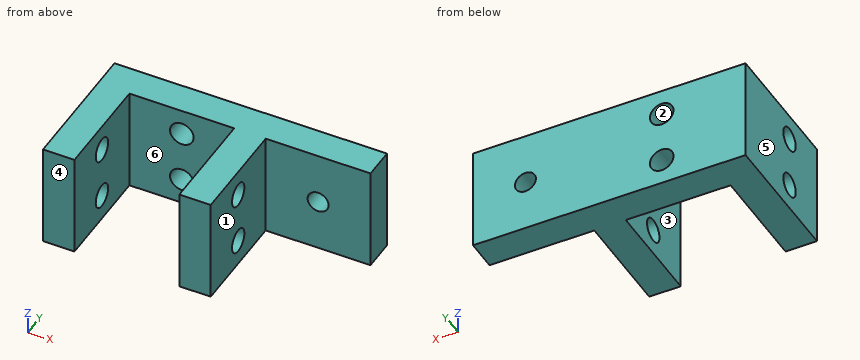
from build123d import *

# Parameters (mm, degrees)
BOSS_EXTRUDE3_DEPTH     = 20
SKETCH9_R               = 2.25
CUT_EXTRUDE1_DEPTH      = 47
CUT_EXTRUDE1_DEPTH_BACK = 7
SKETCH10_R              = 2.25
CUT_EXTRUDE2_DEPTH      = 21
CUT_EXTRUDE2_DEPTH_BACK = 7
SKETCH11_R              = 2
CUT_EXTRUDE3_DEPTH      = 21
CUT_EXTRUDE3_DEPTH_BACK = 7


with BuildPart() as part:
    # Sketch7 → Boss-Extrude3 (new body)
    with BuildSketch(Plane.XY):
        Polygon((-52, -26), (-52, 0), (0, 0), (0, -6), (-20, -6), (-20, -26), (-26, -26), (-26, -6), (-46, -6), (-46, -26), align=None)
    extrude(amount=BOSS_EXTRUDE3_DEPTH)

    # Sketch9 → Cut-Extrude1 (cut, two sides)
    with BuildSketch(Plane(origin=(-46, 0, 0), x_dir=(0, 0, -1), z_dir=(1, 0, 0))) as cut_extrude1_sk:
        with Locations((-15, -16)):
            Circle(SKETCH9_R)
        with Locations((-5, -16)):
            Circle(SKETCH9_R)
    extrude(amount=CUT_EXTRUDE1_DEPTH, mode=Mode.SUBTRACT)
    extrude(cut_extrude1_sk.sketch, amount=-CUT_EXTRUDE1_DEPTH_BACK, mode=Mode.SUBTRACT)

    # Sketch10 → Cut-Extrude2 (cut, two sides)
    with BuildSketch(Plane.XZ.offset(6)) as cut_extrude2_sk:
        with Locations((-36, 5)):
            Circle(SKETCH10_R)
        with Locations((-36, 15)):
            Circle(SKETCH10_R)
    extrude(amount=CUT_EXTRUDE2_DEPTH, mode=Mode.SUBTRACT)
    extrude(cut_extrude2_sk.sketch, amount=-CUT_EXTRUDE2_DEPTH_BACK, mode=Mode.SUBTRACT)

    # Sketch11 → Cut-Extrude3 (cut, two sides)
    with BuildSketch(Plane.XZ.offset(6)) as cut_extrude3_sk:
        with Locations((-10, 10)):
            Circle(SKETCH11_R)
    extrude(amount=CUT_EXTRUDE3_DEPTH, mode=Mode.SUBTRACT)
    extrude(cut_extrude3_sk.sketch, amount=-CUT_EXTRUDE3_DEPTH_BACK, mode=Mode.SUBTRACT)


solid = part.part
The listing builds one solid part. Answer for the finished solid, in the listing's coordinates (mm). Face numbers are marked on the shaded views. A direction names the side the tool comes from. Give positions to 0.01 mm unless a question says otherwise; leave off trailing zeros. Write each loop counter-clockwise with the first axis right and the second up, starting at its lowest first coordinate (ties: lowest second). Pieces come first, ordered by that corner, then holes.
Item 1: Determine the mould class of the marked faces 4, 5 and 6 for opening direction X: released by +X, released by -X, zero draft, split by the parting line, or undercut.
Item 2: Flat-ended cylindrical pins translate along their axes: P1, Ø10, axis at y = -18, z = 9.5, coming from the +X side; P2, Ø3.5, axis at y = -16, z = 5, coming from the -X side; P3, Ø5, axis at x = -6, z = 7, coming from the -Y side. Find the tip coordinate at first contact, or state that the pin passes through.
Item 3: Section B-B, the plane y = -7.25 is taken. Write down the section's boundary in (x, z).
Item 4: Which of the six approach directions +Z, -Z, +X, -X, +Y, -Y give full straight-line access (tool end or side, diameter ignored) to the marked faces 1, 2 and 3?
Item 5: Section C-C, the plane x = -36 is taken. Write down the section's boundary in (y, z).
Item 6: Find the intervals of material crossed by line 1 along Z through (x, y) = (-24.35, -16); line 2 along Y through (x, z) = (-21.85, 5); line 3 along X through (y, z) = (-11, 10), in increasing order.
Item 7: Section D-D, the plane z = 10 is taken. Write down the section's boundary in (x, y).
Item 8: Section A-A, the plane z = 5 is taken. Write down the section's boundary in (x, y).
Completed:
1. face 4: zero draft
1. face 5: released by -X
1. face 6: undercut
2. P1: stops at x = -20
2. P2: passes through
2. P3: stops at y = -6
3. outline: (-52, 0) - (-46, 0) - (-46, 20) - (-52, 20) - close; (-26, 0) - (-20, 0) - (-20, 20) - (-26, 20) - close
4. face 1: +Z, -Z, +X, -Y
4. face 2: +Y, -Y
4. face 3: +Z, -Z, -Y
5. outline: (-6, 0) - (0, 0) - (0, 2.75) - (-6, 2.75) - close; (-6, 7.25) - (0, 7.25) - (0, 12.75) - (-6, 12.75) - close; (-6, 17.25) - (0, 17.25) - (0, 20) - (-6, 20) - close
6. line 1: z = 0 to 2.75, 7.25 to 12.75, 17.25 to 20
6. line 2: y = -26 to -18.25, -13.75 to 0
6. line 3: x = -52 to -46, -26 to -20
7. outline: (-52, -26) - (-46, -26) - (-46, -6) - (-26, -6) - (-26, -26) - (-20, -26) - (-20, -6) - (-12, -6) - (-12, 0) - (-52, 0) - close; (-8, -6) - (0, -6) - (0, 0) - (-8, 0) - close
8. outline: (-52, -26) - (-46, -26) - (-46, -18.25) - (-52, -18.25) - close; (-52, -13.75) - (-46, -13.75) - (-46, -6) - (-38.25, -6) - (-38.25, 0) - (-52, 0) - close; (-33.75, -6) - (-26, -6) - (-26, -13.75) - (-20, -13.75) - (-20, -6) - (0, -6) - (0, 0) - (-33.75, 0) - close; (-26, -26) - (-20, -26) - (-20, -18.25) - (-26, -18.25) - close
